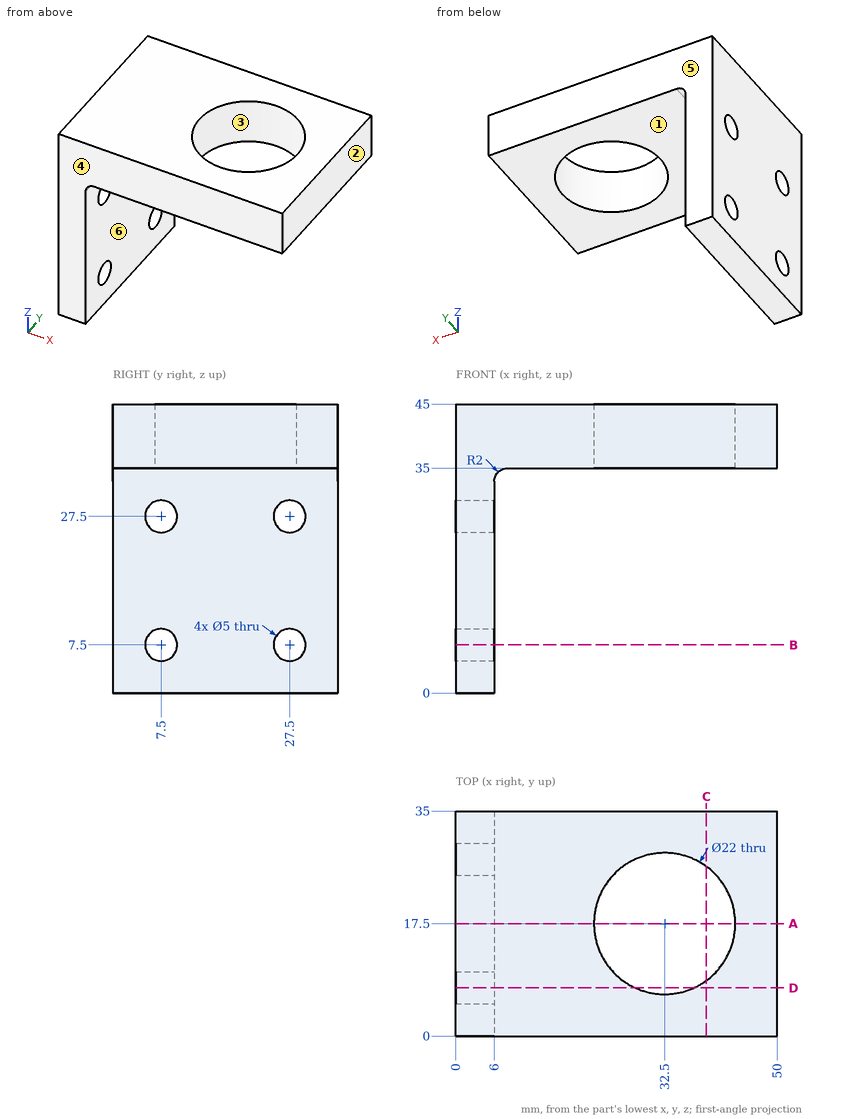
Input: dimensioned drawing with shaded views. Units: mm. Origin: part minimum x, y, z. A direction names the side the tool comes from. Coordinates: 2 decimals unless noted, no trailing zeros. Write each loop counter-clockwise with the first axis right and the second up, starting at its lowest first coordinate (ties: lowest second). Pieces come first, ordered by that corner, then holes. Notation, with made-up numbers: M -5,-21 L 3,-21 A27 cw 3,-2 Z; hole C 4,43 d1. An arc over 180 degrees is marked long. Use one line per item in the form item = value.
Q1. Set-up query: the marked faces 1 and 2. Return all of +Z, -Z, +X, -X, +Y, -Y with unobstructed straight access to the full face (end or side cutting, diameter ignored); none if empty.
Answer below:
face_1 = -Z, +X, +Y, -Y
face_2 = +Z, -Z, +X, +Y, -Y
Q2. First-contact query: pin 1 (4.5 mm diameter, centred on y = 27.5, z = 27.5, fed in from -X); pin 2 (6 mm diameter, centred on y = 7.5, z = 7.5, fed in from +X); pin 3 (2 mm diameter, centred on x = 19, y = 17.5, fed in from -Z). Flat tips, straight axial feed; report the tip coordinate or a pass-through.
Answer below:
pin_1 = through
pin_2 = 6
pin_3 = 35
Q3. Material intervals for probe 1 along Z at (x, y) = (2, 27); probe 2 along Y at (x, z) = (32.5, 38); probe 3 along Y at (x, z) = (3, 7), sorted ascending. Write a range as from..to.
Answer below:
probe_1 = 0..5.05, 9.95..25.05, 29.95..45
probe_2 = 0..6.5, 28.5..35
probe_3 = 0..5.05, 9.95..25.05, 29.95..35
Q4. Section A-A (y = 17.5). Return loops of the section in (x, z), plus the area to 3 significant figures.
Answer below:
outline = M 0,0 L 6,0 L 6,33 A2 cw 8,35 L 21.5,35 L 21.5,45 L 0,45 Z; M 43.5,35 L 50,35 L 50,45 L 43.5,45 Z
area = 491 mm²
Q5. Section D-D (y = 7.5). Return loops of the section in (x, z).
Answer below:
outline = M 0,0 L 6,0 L 6,5 L 0,5 Z; M 0,10 L 6,10 L 6,25 L 0,25 Z; M 0,30 L 6,30 L 6,33 A2 cw 8,35 L 27.92,35 L 27.92,45 L 0,45 Z; M 37.08,35 L 50,35 L 50,45 L 37.08,45 Z
Q6. Section B-B (z = 7.5). Return loops of the section in (x, y), plus the area to 3 significant figures.
Answer below:
outline = M 0,0 L 6,0 L 6,5 L 0,5 Z; M 0,10 L 6,10 L 6,25 L 0,25 Z; M 0,30 L 6,30 L 6,35 L 0,35 Z
area = 150 mm²
Q7. Section C-C (x = 39). Return loops of the section in (y, z), plus the area to 3 significant figures.
Answer below:
outline = M 0,35 L 8.63,35 L 8.63,45 L 0,45 Z; M 26.37,35 L 35,35 L 35,45 L 26.37,45 Z
area = 173 mm²
Q8. Draft query along Y for the marked faces 3, 4, 5 and 6. Return one class per face: released by +Y, released by -Y, zero draft, split by the parting line, or undercut.
Answer below:
face_3 = undercut
face_4 = released by -Y
face_5 = released by +Y
face_6 = zero draft
